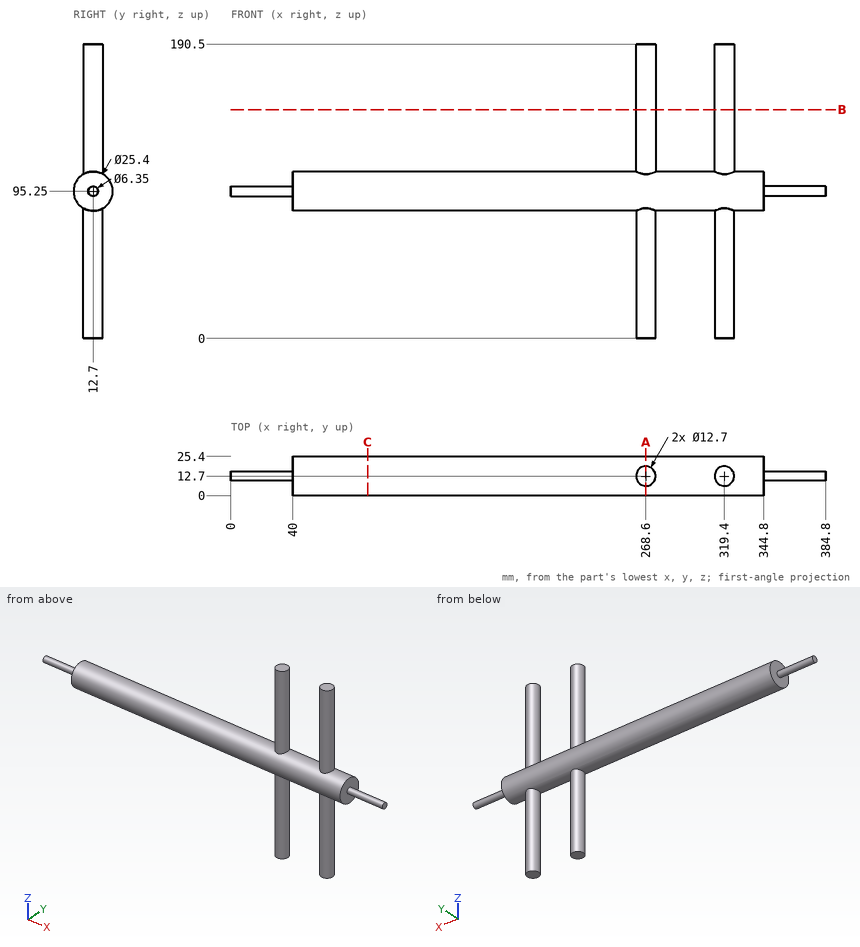
Check sheet for the drawn part. Datum: minimum x, y, z corner. Units: mm. Give positions to 0.01 mm unless a question says otherwise; leave off trailing zeros. Loops run counter-clockwise (first coordinate to the right, second up) from the corner with the lowest first, then second, coordinate; pieces in that order, holes last. Notation, with made-up numbers: M -33.5,86.25 L -2.5,86.25 A12 ccw -2.5,105.25 Z; hole C -18.5,45 d3. An arc over 180 degrees is marked long. Return JSON: item names as keys, results as strings.
1) Section check A-A, the plane x = 268.6. Enter the section's corners in (y, z).
Findings:
{"outline": "M 6.35,0 L 19.05,0 L 19.05,84.25 A12.7 ccw 19.05,106.25 L 19.05,190.5 L 6.35,190.5 L 6.35,106.25 A12.7 ccw 6.35,84.25 Z"}
2) Gauge pin test, flat ends, axial feed: P1, Ø2, axis at x = 51, y = 15.5, coming from the +Z side; P2, Ø4, axis at y = 7, z = 82, coming from the -X side; P3, Ø1, axis at y = 6.5, z = 23, coming from the -X side; P4, Ø10, axis at x = 256, z = 37.5, coming from the +Y side. Record the tip position at first contact, or that the pin passes through.
Findings:
{"P1": "stops at z = 107.82", "P2": "stops at x = 40", "P3": "stops at x = 265.8", "P4": "passes through"}
3) Material ranges on L1, parallel to X at y = 6.5, z = 89; L2, parallel to X at y = 14.5, z = 47.5; L3, parallel to Y at x = 268, z = 150, recorded low to high. Write a range as [from, to].
Findings:
{"L1": "x = [40, 344.8]", "L2": "x = [262.51, 274.69], [313.31, 325.49]", "L3": "y = [6.38, 19.02]"}
4) Section check B-B, the plane z = 148. Enter the section's corners in (x, y), and give its area (3 significant figures).
Findings:
{"outline": "C 268.6,12.7 d12.7; C 319.4,12.7 d12.7", "area": "253 mm2"}
5) Section check C-C, the plane x = 88.5. Enter the section's corners in (y, z).
Findings:
{"outline": "C 12.7,95.25 d25.4"}
